Could you check a few things on this model? Use its own coordinates, in mm. Coordinates: 2 decimals unless noted, no trailing zeros. Loops run counter-clockwise (first coordinate to the right, second up) from the corner with the lowest first, then second, coordinate; pieces in that order, holes last. Notation, with made-up numbers: (-29, -7.75) -> (-18, -7.75) arc R17 cw to (-18, 10.25) -> close; hole circle Ø2 at (52, -30). An arc over 180 degrees is marked (long way). One line per question, with ' | ' between items.
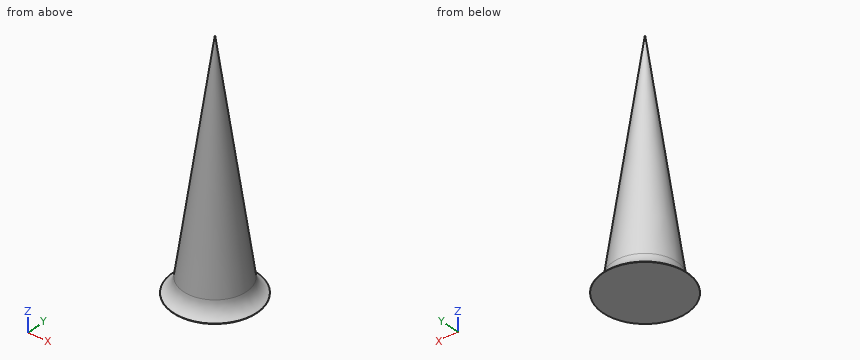
from build123d import *

# Parameters (mm, degrees)
F0_R     = 85
F2_R     = 0.5
F4_R     = 105.9677495378
F5_DEPTH = 1


# Not quite as in the source:
# - a fillet or chamfer that OpenCascade refuses, or shapes differently, is made with other operations: its cross-section is extruded or revolved along the edge and cut away or added


with BuildPart() as f3:
    # F0 (on Top) → F3 section 0
    with BuildSketch(Plane.XY):
        Circle(F0_R)
    # F2 (on offset) → F3 section 1
    with BuildSketch(Plane.XY.offset(600)):
        Circle(F2_R)
    loft()

    # F4 (on Top) → F5 (join)
    with BuildSketch(Plane.XY):
        Circle(F4_R)
    extrude(amount=F5_DEPTH)

    # F6: fillet of radius 50 on 1 edges, made by hand


with BuildPart() as f6_tool2:
    # F6_s3 → F6_t4 (revolve)
    with BuildSketch(Plane.XZ):
        with BuildLine():
            ThreePointArc((105.9675643904, 0.9996454292), (88.2642581979, 16.4841709207), (79.5987288587, 38.349352857))
            Line((79.5987288587, 38.349352857), (74.6474267674, 37.6520444791))
            ThreePointArc((74.6474267674, 37.6520444791), (77.2778437171, 18.9773959421), (79.9078645754, 0.3026916222))
            Line((79.9078645754, 0.3026916222), (84.8591666667, -4.0001631346))
            ThreePointArc((84.8591666667, -4.0001631346), (95.4133655285, -4.0001631346), (103.6531458523, -3.4326336914))
            Line((103.6531458523, -3.4326336914), (105.9675643904, 0.9996454292))
        make_face()
    revolve(axis=Axis((0, 0, 1), (0, 0, 1)))

    split(bisect_by=Plane.XY, keep=Keep.TOP)


with BuildPart() as f3_1:
    add(f3.part)

    # F6_t1: union F6_tool2
    add(f6_tool2.part)


solid = f3_1.part
1) If we section it at B-B on z = 81: Please give me the cut outline in (x, y) (1 decimal).
Data:
outline: circle Ø147.2 at (0, 0)
2) If we section it at A-A on z = 218.5: Please give me the cut outline in (x, y).
Data:
outline: circle Ø108.46 at (0, 0)
3) I need wall thicknesses on line 1 along X through (y, z) = (63, 73.5); line 2 along X through (y, z) = (29.5, 89); line 3 along Y through (x, z) = (47.5, 31). Which ranges of each line are inside material? Lowest first, please. Write a range as from..to.
Data:
line 1: -40.04..40.04 | line 2: -66.19..66.19 | line 3: -65.86..65.86
4) I'm going to push a flat-ended pin straight in: pin 1 Ø5 at (y, z) = (-14.5, 189.5) entering from +X. Where does the tip first touch, or does it pass through?
Data:
pin 1: x = 57.17
